Geometry: see drawing. Coordinates: mm, zero at the bounding-box minimum. A direction names the side the tool comes from. Round coordinates to 2 decimals unless told otherwise and drop trailing zeros. Write each loop counter-clockwise with the first axis right and the second up, starting at its lowest first coordinate (ties: lowest second). Pieces come first, ordered by that corner, then holes. Notation, with made-up numbers: M 84,20 L 119,20 A28 ccw 119,46 Z; hole C 70,77 d11. An arc over 180 degrees is marked long. Write each question's results on one line, items separated by ' | '. Start each with the question number.
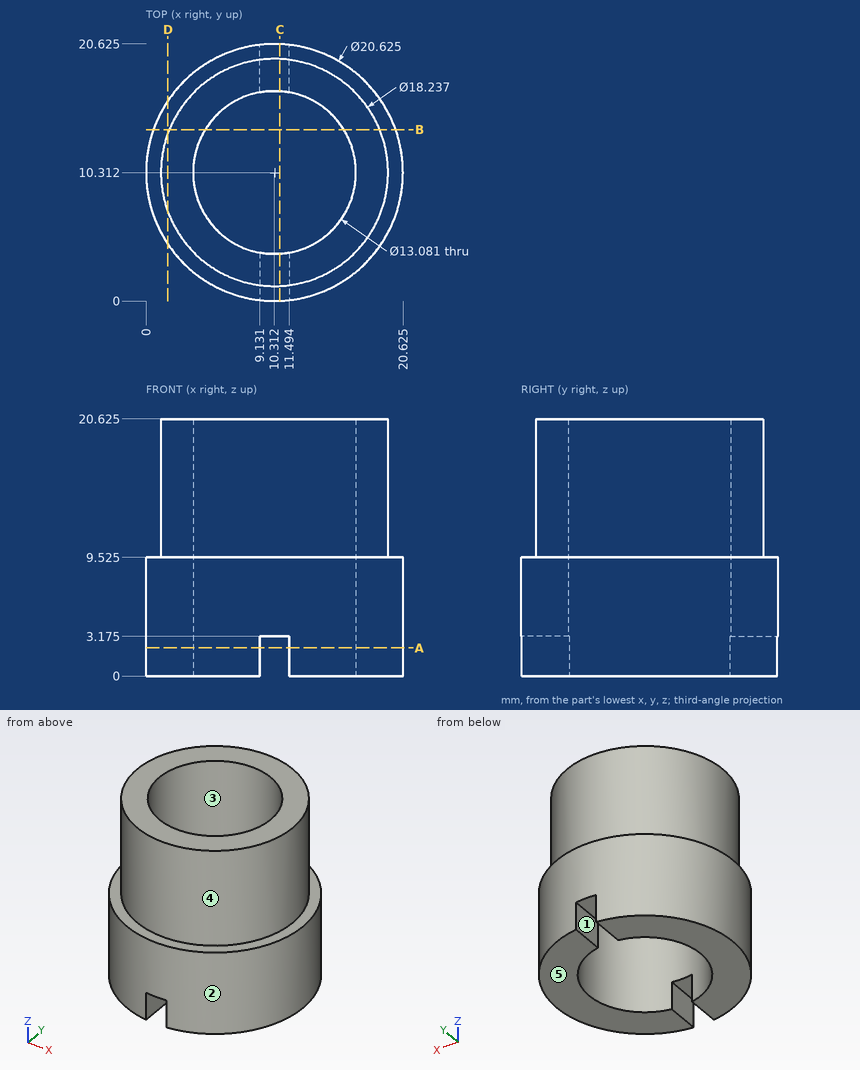
1. Contact query for flat-ended pins moving along their axis: P1, Ø3.5, axis at y = 2, z = 1.5, coming from the -X side; P2, Ø6, axis at x = 10, y = 5.5, coming from the +Z side (1 decimal); P3, Ø10, axis at x = 2, z = 3, coming from the +Y side; P4, Ø1.2, axis at x = 10.5, y = 2, coming from the -Z side (1 decimal). Output: stop coordinate, or through.
2. Cut plane A-A on z = 2.25. Output: boundary loops of the cut face in (x, y) (1 decimal).
3. Draft query along X for the marked faces 3, 4 and 5. Return one class per face: +X half, -X half, draft (parallel to the pull), parting line (faces both ways), or undercut.
4. Cut plane D-D on x = 1.75. Output: boundary loops of the cut face in (y, z) (1 decimal), and give its area (3 significant figures).
5. Access query for the marked faces 1 and 2. Directions: +Z, -Z, +X, -X, +Y, -Y. A direction counts if a zero-diameter tool reaches every point of the face in a straight line with its end or side. Return the directions, or none.
6. Line query: L1, parallel to Z at x = 19.75, y = 11 (1 decimal); L2, parallel to X at y = 16, z = 3.75 (1 decimal); L3, parallel to X at y = 11.5, z = 6.5 (1 decimal). Output: solid intervals per line, ascending. Write a range as from..to.
7. Cut plane C-C on x = 10.75. Output: boundary loops of the cut face in (y, z) (1 decimal), and give its area (3 significant figures).
8. Cut plane B-B on y = 13.75. Output: boundary loops of the cut face in (x, z) (1 decimal).
Answers follow:
1) P1: stops at x = 2.36 | P2: stops at z = 20.6 | P3: stops at y = 20.08 | P4: stops at z = 3.2
2) outline: M 9.1,0.1 L 9.1,3.9 A6.5 cw 9.1,16.7 L 9.1,20.6 A10.3 ccw Z; M 11.5,0.1 A10.3 ccw 11.5,20.6 L 11.5,16.7 A6.5 cw 11.5,3.9 Z
3) face 3: undercut | face 4: parting line | face 5: draft
4) outline: M 4.6,0 L 16.1,0 L 16.1,9.5 L 13.4,9.5 L 13.4,20.6 L 7.2,20.6 L 7.2,9.5 L 4.6,9.5 Z | area: 179 mm2
5) face 1: -Z, +Y, -Y | face 2: +Z, -Z
6) L1: z = 0..9.5 | L2: x = 1.7..7.1, 13.5..18.9 | L3: x = 0.1..3.9, 16.7..20.6
7) outline: M 0,3.2 L 3.8,3.2 L 3.8,20.6 L 1.2,20.6 L 1.2,9.5 L 0,9.5 Z; M 16.8,3.2 L 20.6,3.2 L 20.6,9.5 L 19.4,9.5 L 19.4,20.6 L 16.8,20.6 Z | area: 105 mm2
8) outline: M 0.6,0 L 4.7,0 L 4.7,20.6 L 1.9,20.6 L 1.9,9.5 L 0.6,9.5 Z; M 15.9,0 L 20,0 L 20,9.5 L 18.8,9.5 L 18.8,20.6 L 15.9,20.6 Z
